from build123d import *

# Parameters (mm, degrees)
F0_W         = 80
F0_H         = 35
F0_W_2       = 60
F0_H_2       = 10
F0_W_3       = 3
F1_DEPTH     = 3
F2_DEPTH     = 12.525
F3_DEPTH     = 7.968
F4_DEPTH     = 23
F5_R         = 1.5
F6_DEPTH     = 128.501
F7_T1_DEPTH  = 60
F7_T3_DEPTH  = 47.5
F7_T5_DEPTH  = 20.5
F7_T7_DEPTH  = 32.5
F7_T9_DEPTH  = 20.5
F7_T11_DEPTH = 47.5
F7_T16_ANGLE = 130.941996925
F7_T22_ANGLE = 130.941996925
F7_T26_ANGLE = 94.0941996925
F7_T28_ANGLE = 94.0941996925
F7_T30_ANGLE = 90
F7_T32_ANGLE = 90


# Not quite as in the source:
# - a fillet or chamfer that OpenCascade refuses, or shapes differently, is made with other operations: its cross-section is extruded or revolved along the edge and cut away or added


with BuildPart() as f1:
    # F0 (on Top) → F1 (new body)
    with BuildSketch(Plane.XY):
        with Locations((0, -17.5)):
            Rectangle(F0_W, F0_H)
        with BuildLine():
            Line((-88.5, 35), (-88.5, 0))
            ThreePointArc((-88.5, 0), (-78.2487373415, 24.7487373415), (-53.5, 35))
            Line((-53.5, 35), (-88.5, 35))
        make_face()
        with BuildLine():
            ThreePointArc((53.5, 35), (78.2487373415, 24.7487373415), (88.5, 0))
            Line((88.5, 0), (88.5, 35))
            Line((88.5, 35), (53.5, 35))
        make_face()
        with BuildLine():
            Line((-95.5, 30), (-95.5, 0))
            Line((-95.5, 0), (-88.5, 0))
            Line((-88.5, 0), (-88.5, 35))
            Line((-88.5, 35), (-53.5, 35))
            Line((-53.5, 35), (-33, 35))
            Line((-33, 35), (-33, 45))
            Line((-33, 45), (-80.5, 45))
            ThreePointArc((-80.5, 45), (-91.1066017178, 40.6066017178), (-95.5, 30))
        make_face()
        with Locations((0, 40)):
            Rectangle(F0_W_2, F0_H_2)
        with BuildLine():
            Line((88.5, 35), (88.5, 0))
            Line((88.5, 0), (95.5, 0))
            Line((95.5, 0), (95.5, 30))
            ThreePointArc((95.5, 30), (91.1066017178, 40.6066017178), (80.5, 45))
            Line((80.5, 45), (33, 45))
            Line((33, 45), (33, 35))
            Line((33, 35), (53.5, 35))
            Line((53.5, 35), (88.5, 35))
        make_face()
        with Locations((-31.5, 40)):
            Rectangle(F0_W_3, F0_H_2)
        with Locations((31.5, 40)):
            Rectangle(F0_W_3, F0_H_2)
        with BuildLine():
            ThreePointArc((-53.5, 35), (-78.2487373415, 24.7487373415), (-88.5, 0))
            Line((-88.5, 0), (-40, 0))
            Line((-40, 0), (40, 0))
            Line((40, 0), (88.5, 0))
            ThreePointArc((88.5, 0), (78.2487373415, 24.7487373415), (53.5, 35))
            Line((53.5, 35), (33, 35))
            Line((33, 35), (30, 35))
            Line((30, 35), (-30, 35))
            Line((-30, 35), (-33, 35))
            Line((-33, 35), (-53.5, 35))
        make_face()
    extrude(amount=-F1_DEPTH)

    # F0 (on Top) → F2 (join)
    with BuildSketch(Plane.XY):
        with BuildLine():
            Line((-95.5, 30), (-95.5, 0))
            Line((-95.5, 0), (-88.5, 0))
            Line((-88.5, 0), (-88.5, 35))
            Line((-88.5, 35), (-53.5, 35))
            Line((-53.5, 35), (-33, 35))
            Line((-33, 35), (-33, 45))
            Line((-33, 45), (-80.5, 45))
            ThreePointArc((-80.5, 45), (-91.1066017178, 40.6066017178), (-95.5, 30))
        make_face()
        with Locations((-31.5, 40)):
            Rectangle(F0_W_3, F0_H_2)
        with Locations((0, 40)):
            Rectangle(F0_W_2, F0_H_2)
        with Locations((31.5, 40)):
            Rectangle(F0_W_3, F0_H_2)
        with BuildLine():
            Line((88.5, 35), (88.5, 0))
            Line((88.5, 0), (95.5, 0))
            Line((95.5, 0), (95.5, 30))
            ThreePointArc((95.5, 30), (91.1066017178, 40.6066017178), (80.5, 45))
            Line((80.5, 45), (33, 45))
            Line((33, 45), (33, 35))
            Line((33, 35), (53.5, 35))
            Line((53.5, 35), (88.5, 35))
        make_face()
        with BuildLine():
            Line((-88.5, 35), (-88.5, 0))
            ThreePointArc((-88.5, 0), (-78.2487373415, 24.7487373415), (-53.5, 35))
            Line((-53.5, 35), (-88.5, 35))
        make_face()
        with BuildLine():
            ThreePointArc((53.5, 35), (78.2487373415, 24.7487373415), (88.5, 0))
            Line((88.5, 0), (88.5, 35))
            Line((88.5, 35), (53.5, 35))
        make_face()
    extrude(amount=F2_DEPTH)

    # F0 (on Top) → F3 (cut)
    with BuildSketch(Plane.XY):
        with BuildLine():
            Line((-88.5, 35), (-88.5, 0))
            ThreePointArc((-88.5, 0), (-78.2487373415, 24.7487373415), (-53.5, 35))
            Line((-53.5, 35), (-88.5, 35))
        make_face()
        with BuildLine():
            ThreePointArc((53.5, 35), (78.2487373415, 24.7487373415), (88.5, 0))
            Line((88.5, 0), (88.5, 35))
            Line((88.5, 35), (53.5, 35))
        make_face()
    extrude(amount=F3_DEPTH, mode=Mode.SUBTRACT)

    # F0 (on Top) → F4 (join)
    with BuildSketch(Plane.XY):
        with Locations((-31.5, 40)):
            Rectangle(F0_W_3, F0_H_2)
        with Locations((31.5, 40)):
            Rectangle(F0_W_3, F0_H_2)
    extrude(amount=F4_DEPTH)

    # F5 (on face) → F6 (cut, through all)
    with BuildSketch(Plane(origin=(-33, 0, 0), x_dir=(0, -1, 0), z_dir=(-1, 0, 0))):
        with Locations((-40, 17.7625)):
            Circle(F5_R)
    extrude(amount=-F6_DEPTH, mode=Mode.SUBTRACT)

    # F7: fillet of radius 1 on 14 edges, made by hand

    # F7_s2 → F7_t1 (cut)
    with BuildSketch(Plane.YZ.offset(-30)):
        with BuildLine():
            ThreePointArc((45, 11.525), (44.7071067812, 12.2321067812), (44, 12.525))
            Line((44, 12.525), (45, 12.525))
            Line((45, 12.525), (45, 11.525))
        make_face()
        with BuildLine():
            ThreePointArc((35, 11.525), (35.2928932188, 12.2321067812), (36, 12.525))
            Line((36, 12.525), (35, 12.525))
            Line((35, 12.525), (35, 11.525))
        make_face()
    extrude(amount=F7_T1_DEPTH, mode=Mode.SUBTRACT)

    # F7_s4 → F7_t3 (cut)
    with BuildSketch(Plane.YZ.offset(-80.5)):
        with BuildLine():
            ThreePointArc((44, 12.525), (44.7071067812, 12.2321067812), (45, 11.525))
            Line((45, 11.525), (45, 12.525))
            Line((45, 12.525), (44, 12.525))
        make_face()
    extrude(amount=F7_T3_DEPTH, mode=Mode.SUBTRACT)

    # F7_s6 → F7_t5 (cut)
    with BuildSketch(Plane.YZ.offset(-53.5)):
        with BuildLine():
            ThreePointArc((36, 12.525), (35.2928932188, 12.2321067812), (35, 11.525))
            Line((35, 11.525), (35, 12.525))
            Line((35, 12.525), (36, 12.525))
        make_face()
    extrude(amount=F7_T5_DEPTH, mode=Mode.SUBTRACT)

    # F7_s8 → F7_t7 (cut)
    with BuildSketch(Plane.XZ.offset(-30)):
        with BuildLine():
            ThreePointArc((-94.5, 12.525), (-95.2071067812, 12.2321067812), (-95.5, 11.525))
            Line((-95.5, 11.525), (-95.5, 12.525))
            Line((-95.5, 12.525), (-94.5, 12.525))
        make_face()
        with BuildLine():
            ThreePointArc((95.5, 11.525), (95.2071067812, 12.2321067812), (94.5, 12.525))
            Line((94.5, 12.525), (95.5, 12.525))
            Line((95.5, 12.525), (95.5, 11.525))
        make_face()
    extrude(amount=F7_T7_DEPTH, mode=Mode.SUBTRACT)

    # F7_s10 → F7_t9 (cut)
    with BuildSketch(Plane.YZ.offset(33)):
        with BuildLine():
            ThreePointArc((35, 11.525), (35.2928932188, 12.2321067812), (36, 12.525))
            Line((36, 12.525), (35, 12.525))
            Line((35, 12.525), (35, 11.525))
        make_face()
    extrude(amount=F7_T9_DEPTH, mode=Mode.SUBTRACT)

    # F7_s12 → F7_t11 (cut)
    with BuildSketch(Plane.YZ.offset(33)):
        with BuildLine():
            ThreePointArc((45, 11.525), (44.7071067812, 12.2321067812), (44, 12.525))
            Line((44, 12.525), (45, 12.525))
            Line((45, 12.525), (45, 11.525))
        make_face()
    extrude(amount=F7_T11_DEPTH, mode=Mode.SUBTRACT)


with BuildPart() as f7_tool14:
    # F7_s15 → F7_t16 (revolve)
    with BuildSketch(Plane(origin=(-6.5437628549, 17.5291323355, 0), x_dir=(0, 0, 1), z_dir=(0.3497332189, -0.9368493345, 0))):
        with BuildLine():
            ThreePointArc((8.968, 85.1214393974), (8.2608932188, 85.4143326162), (7.968, 86.1214393974))
            Line((7.968, 86.1214393974), (7.968, 85.1214393974))
            Line((7.968, 85.1214393974), (8.968, 85.1214393974))
        make_face()
    revolve(axis=Axis((-53.5, 0, 7.968), (0, 0, -1)), revolution_arc=F7_T16_ANGLE)

    split(bisect_by=Plane.YZ.offset(-88.5), keep=Keep.TOP)

    split(bisect_by=Plane.XZ.offset(-35), keep=Keep.TOP)


with BuildPart() as f1_1:
    add(f1.part)

    # F7_t13: cut F7_tool14
    add(f7_tool14.part, mode=Mode.SUBTRACT)


with BuildPart() as f7_tool20:
    # F7_s21 → F7_t22 (revolve)
    with BuildSketch(Plane(origin=(46.9562371451, 17.5291323355, 0), x_dir=(0, 0, 1), z_dir=(-0.9368493345, -0.3497332189, 0))):
        with BuildLine():
            ThreePointArc((8.968, 16.2892727897), (8.2608932188, 16.5821660086), (7.968, 17.2892727897))
            Line((7.968, 17.2892727897), (7.968, 16.2892727897))
            Line((7.968, 16.2892727897), (8.968, 16.2892727897))
        make_face()
    revolve(axis=Axis((53.5, 0, 7.968), (0, 0, -1)), revolution_arc=F7_T22_ANGLE)

    split(bisect_by=Plane.YZ.offset(88.5), keep=Keep.BOTTOM)

    split(bisect_by=Plane.XZ.offset(-35), keep=Keep.TOP)


with BuildPart() as f1_2:
    add(f1_1.part)

    # F7_t19: cut F7_tool20
    add(f7_tool20.part, mode=Mode.SUBTRACT)

    # F7_s25 → F7_t26 (revolve, cut)
    with BuildSketch(Plane(origin=(-0.2727138814, 3.809963227, 0), x_dir=(0, 0, 1), z_dir=(0.0713964686, -0.9974480158, 0))):
        with BuildLine():
            ThreePointArc((11.525, 88.3634688467), (12.2321067812, 88.6563620655), (12.525, 89.3634688467))
            Line((12.525, 89.3634688467), (12.525, 88.3634688467))
            Line((12.525, 88.3634688467), (11.525, 88.3634688467))
        make_face()
    revolve(axis=Axis((-53.5, 0, 12.525), (0, 0, -1)), revolution_arc=F7_T26_ANGLE, mode=Mode.SUBTRACT)

    # F7_s27 → F7_t28 (revolve, cut)
    with BuildSketch(Plane.YZ.offset(53.5)):
        with BuildLine():
            ThreePointArc((36, 12.525), (35.2928932188, 12.2321067812), (35, 11.525))
            Line((35, 11.525), (35, 12.525))
            Line((35, 12.525), (36, 12.525))
        make_face()
    revolve(axis=Axis((53.5, 0, 12.525), (0, 0, -1)), revolution_arc=F7_T28_ANGLE, mode=Mode.SUBTRACT)

    # F7_s29 → F7_t30 (revolve, cut)
    with BuildSketch(Plane.XZ.offset(-30)):
        with BuildLine():
            ThreePointArc((95.5, 11.525), (95.2071067812, 12.2321067812), (94.5, 12.525))
            Line((94.5, 12.525), (95.5, 12.525))
            Line((95.5, 12.525), (95.5, 11.525))
        make_face()
    revolve(axis=Axis((80.5, 30, 12.525), (0, 0, 1)), revolution_arc=F7_T30_ANGLE, mode=Mode.SUBTRACT)

    # F7_s31 → F7_t32 (revolve, cut)
    with BuildSketch(Plane.YZ.offset(-80.5)):
        with BuildLine():
            ThreePointArc((44, 12.525), (44.7071067812, 12.2321067812), (45, 11.525))
            Line((45, 11.525), (45, 12.525))
            Line((45, 12.525), (44, 12.525))
        make_face()
    revolve(axis=Axis((-80.5, 30, 12.525), (0, 0, 1)), revolution_arc=F7_T32_ANGLE, mode=Mode.SUBTRACT)


solid = f1_2.part
Part model, mm, in its own coordinate system. A direction names the side the tool comes from. Give positions to 0.01 mm unless a question says otherwise; leave off trailing zeros. Write each loop counter-clockwise with the first axis right and the second up, starting at its lowest first coordinate (ties: lowest second). Pieces come first, ordered by that corner, then holes.
1) Which spindle directions (+Z, -Z, +X, -X, +Y, -Y) get a long thin tool onto all of the face, cutting with end or side? Do faces 5 (the face through (-76, 0, -1)), 6 (the face through (-78.519, 24.475, 10.229)), 7 (the face through (-71, 32, 12.525)), 8 (the face through (81, 28, 7.968)). Say none if no direction does.
Resolved:
face 5: +Z, -Z, -X, -Y
face 6: +Z, -Y
face 7: +Z, -X, +Y, -Y
face 8: -Y
2) Cut at A-A on x = -20. Write the cut outline in (y, z) (3 decimals), then the cut area to 3 significant figures.
Resolved:
outline: (-35, -3) - (45, -3) - (45, 11.525) arc R1 ccw to (44, 12.525) - (36, 12.525) arc R1 ccw to (35, 11.525) - (35, 0) - (-35, 0) - close
area: 365 mm2
3) Probe L1, parallel to X at y = 9, z = 6.5; L2, parallel to X at y = 35.5, z = 16; L3, parallel to Z at x = 31.05, y = 40. List the from-to ranges inside material, lowest first.
Resolved:
L1: x = -95.5 to -88.5, 88.5 to 95.5
L2: x = -33 to -30, 30 to 33
L3: z = -3 to 16.26, 19.26 to 23
4) Pin check, flat tips, straight feed: pin 1 (10 mm diameter, centred on y = -6, z = -0.5, fed in from -X); pin 2 (10 mm diameter, centred on x = 31, z = 20, fed in from -Y); pin 3 (3 mm diameter, centred on y = 39.5, z = 16, fed in from +X). Stop position of each tip, or through.
Resolved:
pin 1: stops at x = -40
pin 2: stops at y = 35
pin 3: stops at x = 33
5) Cut at B-B on y = -3. Write the cut outline in (x, z).
Resolved:
outline: (-40, -3) - (40, -3) - (40, 0) - (-40, 0) - close
6) Two-plate mould, pull along Z, no slides. Class faces 1 (the face through (-1, 14, -3)), 2 (the face through (88.5, 17, 5)), 3 (the face through (75.8, 0, -0.4)), 4 (the face through (75, 34, 12.525)): released by +Z, released by -Z, zero draft, split by the parting line, or undercut.
Resolved:
face 1: released by -Z
face 2: undercut
face 3: zero draft
face 4: released by +Z
